Verification items for the finished model (mm, model axes). A direction names the side the tool comes from. Give positions to 0.01 mm unless a question says otherwise; leave off trailing zeros. Write each loop counter-clockwise with the first axis right and the second up, starting at its lowest first coordinate (ties: lowest second). Pieces come first, ordered by that corner, then holes. Notation, with made-up numbers: M 38,-10.75 L 43,-10.75 A25 cw 43,9.25 Z; hole C 21.25,-23 d1. An arc over 180 degrees is marked long. Write item = value, one per line.
from build123d import *

# Parameters (mm, degrees)
F0_W     = 20
F0_H     = 20
F1_DEPTH = 26
F2_W     = 12
F2_H     = 18
F3_DEPTH = 12
F4_W     = 18
F4_H     = 4
F5_DEPTH = 18
F6_W     = 4
F6_H     = 18
F7_DEPTH = 12
F9_DEPTH = 18


with BuildPart() as f1:
    # F0 (on Top) → F1 (new body)
    with BuildSketch(Plane.XY):
        with Locations((10, 10)):
            Rectangle(F0_W, F0_H)
    extrude(amount=F1_DEPTH)

    # F2 (on face) → F3 (cut)
    with BuildSketch(Plane(origin=(0, 0, 0), x_dir=(0, -1, 0), z_dir=(-1, 0, 0))):
        with Locations((-6, 17)):
            Rectangle(F2_W, F2_H)
    extrude(amount=-F3_DEPTH, mode=Mode.SUBTRACT)

    # F4 (on face) → F5 (cut)
    with BuildSketch(Plane(origin=(0, 0, 0), x_dir=(0, -1, 0), z_dir=(-1, 0, 0))):
        with Locations((-9, 4)):
            Rectangle(F4_W, F4_H)
    extrude(amount=-F5_DEPTH, mode=Mode.SUBTRACT)

    # F6 (on face) → F7 (cut)
    with BuildSketch(Plane(origin=(0, 0, 0), x_dir=(0, -1, 0), z_dir=(-1, 0, 0))):
        with Locations((-16, 17)):
            Rectangle(F6_W, F6_H)
    extrude(amount=-F7_DEPTH, mode=Mode.SUBTRACT)

    # F8 (on face) → F9 (cut)
    with BuildSketch(Plane.XY.offset(26)):
        Polygon((12, 18), (12, 14), (16, 18), align=None)
        Polygon((18, 16), (14, 12), (14, 0), (18, 0), (18, 12), align=None)
    extrude(amount=-F9_DEPTH, mode=Mode.SUBTRACT)


solid = f1.part
1) Cross-section at B-B on z = 5. Record the boundary of the cut face in (x, y).
From the geometry:
outline = M 0,18 L 18,18 L 18,0 L 20,0 L 20,20 L 0,20 Z
2) Depth check by flat-ended pin: P1, Ø1.2, axis at y = 11, z = 4.5, coming from the -X side; P2, Ø6, axis at x = 3.5, y = 6.5, coming from the +Z side; P3, Ø5, axis at x = 7.5, z = 14, coming from the -Y side. Enter the tip coordinate at first touch or a pass-through.
From the geometry:
P1 = 18
P2 = 8
P3 = 12
3) Material ranges on probe 1 along X at (y, z) = (7.75, 12); probe 2 along Z at (x, y) = (1.5, 17), recorded low to high. Write a range as from..to.
From the geometry:
probe_1 = 12..14, 18..20
probe_2 = 0..2, 6..8
4) Cross-section at A-A on y = 9.5. Record the boundary of the cut face in (x, z), plus the area to 3 significant figures.
From the geometry:
outline = M 0,0 L 20,0 L 20,26 L 18,26 L 18,8 L 14,8 L 14,26 L 12,26 L 12,8 L 0,8 L 0,6 L 18,6 L 18,2 L 0,2 Z
area = 160 mm^2
5) Draft check along X on faces 4 (the flat face through (12.1, 12.4, 26)), 5 (the flat face through (14, 6, 17)), 6 (the flat face through (0, 12, 7)), 7 (the flat face through (18, 8, 17)). Enter one of: +X half, -X half, draft (parallel to the pull), parting line (faces both ways), or undercut.
From the geometry:
face_4 = draft
face_5 = undercut
face_6 = -X half
face_7 = undercut
6) Cross-section at D-D on y = 12.5. Record the boundary of the cut face in (x, z).
From the geometry:
outline = M 0,0 L 20,0 L 20,26 L 18,26 L 18,8 L 14.5,8 L 14.5,26 L 0,26 L 0,6 L 18,6 L 18,2 L 0,2 Z
7) Tool access check on faces 1 (the flat face through (12, 6, 17)), 2 (the flat face through (16, 6, 8)), 3 (the flat face through (8, 18, 17)). Record the directions out of +Z, -Z, +X, -X, +Y, -Y that give a thin tool (end or side, any length) a straight path to the whole face; none if there is none.
From the geometry:
face_1 = +Z, -X, -Y
face_2 = +Z, -Y
face_3 = +Z, -X
